```python
from build123d import *

# Parameters (mm, degrees)
SKETCH1_W                                         = 355.6
SKETCH1_H                                         = 114.3
SKETCH1_R                                         = 2.15265
SKETCH1_W_2                                       = 6.35
SKETCH1_H_2                                       = 6.604
BOSS_EXTRUDE1_DEPTH                               = 6.604
CUT_EXTRUDE1_DEPTH                                = 7.604
SKETCH6_W                                         = 6.35
SKETCH6_H                                         = 6.35
BOSS_EXTRUDE2_DEPTH                               = 6.604
CSK_FOR_8_FLAT_HEAD_SOCKET_CAP_SCREW1_D           = 4.3053
CSK_FOR_8_FLAT_HEAD_SOCKET_CAP_SCREW1_CSINK_D     = 9.1186
CSK_FOR_8_FLAT_HEAD_SOCKET_CAP_SCREW1_CSINK_ANGLE = 82
F_8_32_TAPPED_HOLE1_D                             = 3.4544
F_8_32_TAPPED_HOLE1_DEPTH                         = 10.7188
F_8_32_TAPPED_HOLE1_TIP                           = 1.037806461


with BuildPart() as part:
    # Sketch1 → Boss-Extrude1 (new body)
    with BuildSketch(Plane(origin=(0, 0, 0), x_dir=(0, 0, -1), z_dir=(1, 0, 0))):
        with Locations((0, 57.15)):
            Rectangle(SKETCH1_W, SKETCH1_H)
        with Locations((-152.4, 9.525)):
            Circle(SKETCH1_R, mode=Mode.SUBTRACT)
        with Locations((0, 9.525)):
            Circle(SKETCH1_R, mode=Mode.SUBTRACT)
        with Locations((152.4, 9.525)):
            Circle(SKETCH1_R, mode=Mode.SUBTRACT)
        with Locations((-142.875, 9.525)):
            Rectangle(SKETCH1_W_2, SKETCH1_H_2, mode=Mode.SUBTRACT)
        with Locations((-161.925, 9.525)):
            Rectangle(SKETCH1_W_2, SKETCH1_H_2, mode=Mode.SUBTRACT)
        with Locations((9.525, 9.525)):
            Rectangle(SKETCH1_W_2, SKETCH1_H_2, mode=Mode.SUBTRACT)
        with Locations((-9.525, 9.525)):
            Rectangle(SKETCH1_W_2, SKETCH1_H_2, mode=Mode.SUBTRACT)
        with Locations((161.925, 9.525)):
            Rectangle(SKETCH1_W_2, SKETCH1_H_2, mode=Mode.SUBTRACT)
        with Locations((142.875, 9.525)):
            Rectangle(SKETCH1_W_2, SKETCH1_H_2, mode=Mode.SUBTRACT)
    extrude(amount=BOSS_EXTRUDE1_DEPTH)

    # Sketch5 → Cut-Extrude1 (cut, through all)
    with BuildSketch(Plane.ZY):
        Polygon((177.8, 90.9828), (171.45, 90.9828), (171.45, 93.2688), (165.5064, 93.2688), (165.5064, 90.9828), (163.83, 90.9828), (163.83, 86.8172), (165.5064, 86.8172), (165.5064, 84.5312), (171.45, 84.5312), (171.45, 86.8172), (177.8, 86.8172), align=None)
    extrude(amount=-CUT_EXTRUDE1_DEPTH, mode=Mode.SUBTRACT)

    # Sketch6 → Boss-Extrude2 (add)
    with BuildSketch(Plane.ZY):
        with Locations((180.975, 98.425)):
            Rectangle(SKETCH6_W, SKETCH6_H)
        with Locations((180.975, 79.375)):
            Rectangle(SKETCH6_W, SKETCH6_H)
    extrude(amount=-BOSS_EXTRUDE2_DEPTH)

    # CSK for #8 Flat Head Socket Cap Screw1 (through all)
    with Locations(Plane.ZY):
        with Locations((-152.4, 9.525), (0, 9.525), (152.4, 9.525)):
            CounterSinkHole(CSK_FOR_8_FLAT_HEAD_SOCKET_CAP_SCREW1_D / 2, CSK_FOR_8_FLAT_HEAD_SOCKET_CAP_SCREW1_CSINK_D / 2, counter_sink_angle=CSK_FOR_8_FLAT_HEAD_SOCKET_CAP_SCREW1_CSINK_ANGLE)

    # #8-32 Tapped Hole1
    with Locations(Plane.ZY):
        with Locations((117.475, 19.05), (-31.75, 19.05)):
            Hole(F_8_32_TAPPED_HOLE1_D / 2, depth=F_8_32_TAPPED_HOLE1_DEPTH)
            with Locations((0, 0, -(F_8_32_TAPPED_HOLE1_DEPTH + F_8_32_TAPPED_HOLE1_TIP / 2))):  # 118° drill point
                Cone(0, F_8_32_TAPPED_HOLE1_D / 2, F_8_32_TAPPED_HOLE1_TIP, mode=Mode.SUBTRACT)


solid = part.part
```
Build history of the part. All positions in model axes, mm. A direction names the side the tool comes from. Round coordinates to 2 decimals unless told otherwise and drop trailing zeros. Use a Markdown table: item, result.
1) Wall check: L1, parallel to Y at x = 5.35, z = 0; L2, parallel to Y at x = 3.5, z = -140; L3, parallel to Z at x = 3, y = 94. Give the ranges that are in metal, low to high.
Recorded:
| item | result |
|---|---|
| L1 | y = 0 to 7.37, 11.68 to 114.3 |
| L2 | y = 0 to 6.22, 12.83 to 114.3 |
| L3 | z = -177.8 to 177.8 |
2) Pull direction Y, two halves, no side cores. Call faces 1 (the face through (3, 114.3, 2)), 2 (the face through (3, 84.531, 168)), 3 (the face through (3, 9, 139.7)), 4 (the face through (3, 108, 177.8)): pulls with the +Y half, pulls with the -Y half, needs draft (parallel to the pull), parting line crosses it, or undercut.
Recorded:
| item | result |
|---|---|
| face 1 | pulls with the +Y half |
| face 2 | undercut |
| face 3 | undercut |
| face 4 | needs draft |
3) Flat gauge pins, fed straight in: pin 1 Ø7 at (y, z) = (9.525, -152.4) entering from -X; pin 2 Ø1.2 at (x, y) = (3, 89) entering from +Z; pin 3 Ø3 at (y, z) = (15, -138) entering from -X; pin 4 Ø1.3 at (x, y) = (4.5, 84) entering from +Z. Where does each tip first touch, or does it go through?
Recorded:
| item | result |
|---|---|
| pin 1 | stops at x = 1.22 |
| pin 2 | stops at z = 163.83 |
| pin 3 | stops at x = 0 |
| pin 4 | stops at z = 177.8 |
4) Tool access for faces 5 (the face through (3, 12.827, 10)), 6 (the face through (3, 56, -177.8)), 7 (the face through (3, 95.25, 181)): list every direction of +Z, -Z, +X, -X, +Y, -Y with a clear straight run to the whole face (end or side of a thin tool).
Recorded:
| item | result |
|---|---|
| face 5 | +X, -X |
| face 6 | -Z, +X, -X, +Y, -Y |
| face 7 | +Z, +X, -X |
5) Saw through at A-A on x = 1.25. Give the number of separate pieces and of enclosed holes in the cut face, and give its area (3 significant figures).
Recorded:
| item | result |
|---|---|
| separate pieces | 1 |
| enclosed holes | 11 |
| area | 40,300 mm² |
